Source: CAD feature listing. Evaluate the final solid. Frame: model axes, mm. A direction names the side the tool comes from. Give positions to 0.01 mm unless a question says otherwise; leave off trailing zeros. Write each loop counter-clockwise with the first axis right and the second up, starting at its lowest first coordinate (ties: lowest second). Pieces come first, ordered by that corner, then holes. Notation, with made-up numbers: (44, 9.25) -> (63, 9.25) arc R18 cw to (63, 42.25) -> close; hole circle Ø11 at (36.25, 76). An arc over 180 degrees is marked (long way). Write item = value, one per line.
from build123d import *

# Parameters (mm, degrees)
BOSS_EXTRUDE1_DEPTH             = 57.5
CUT_EXTRUDE1_DEPTH              = 334.110342079
CUT_EXTRUDE4_START              = 2.5
CUT_EXTRUDE4_DEPTH              = 322.334448445
BOSS_EXTRUDE2_REACH             = 325.834
SKETCH9_R                       = 5
BOSS_EXTRUDE2_DIRECTION_2_REACH = 325.834
CUT_EXTRUDE5_DEPTH              = 324.834448483
CUT_EXTRUDE5_DEPTH_BACK         = 324.834448483
SKETCH9_3_R                     = 5


with BuildPart() as part:
    # Sketch3 → Boss-Extrude1 (new, symmetric)
    with BuildSketch(Plane.YZ):
        with BuildLine():
            Line((242.818015058, -8.927876097), (206.857769199, 33.927876097))
            ThreePointArc((206.857769199, 33.927876097), (203.423507385, 36.56307787), (199.197324767, 37.5))
            Line((199.197324767, 37.5), (-37.5, 37.5))
            Line((-37.5, 37.5), (-37.5, -37.5))
            Line((-37.5, -37.5), (83.860297657, -37.5))
            ThreePointArc((83.860297657, -37.5), (87.280499091, -36.896926208), (90.288173754, -35.160444431))
            Line((90.288173754, -35.160444431), (126.423201987, -4.839555569))
            ThreePointArc((126.423201987, -4.839555569), (129.43087665, -3.103073792), (132.851078083, -2.5))
            Line((132.851078083, -2.5), (167.490945548, -2.5))
            ThreePointArc((167.490945548, -2.5), (171.717128165, -3.43692213), (175.151389979, -6.072123903))
            Line((175.151389979, -6.072123903), (219.50263215, -58.927876097))
            ThreePointArc((219.50263215, -58.927876097), (222.936893964, -61.56307787), (227.163076582, -62.5))
            Line((227.163076582, -62.5), (312.5, -62.5))
            Line((312.5, -62.5), (312.5, -12.5))
            Line((312.5, -12.5), (250.478459489, -12.5))
            ThreePointArc((250.478459489, -12.5), (246.252276872, -11.56307787), (242.818015058, -8.927876097))
        make_face()
    extrude(amount=BOSS_EXTRUDE1_DEPTH, both=True)

    # Sketch4 → Cut-Extrude1 (cut, through all)
    with BuildSketch(Plane.XY.offset(37.5)):
        Polygon((57.5, -37.5), (57.5, 37.5), (0, -37.5), align=None)
        Polygon((0, -37.5), (-57.5, 37.5), (-57.5, -37.5), align=None)
        Polygon((-37.232627886, 27.5), (0, -21.064297242), (0, 27.5), align=None)
        Polygon((0, 27.5), (0, -21.064297242), (37.232627886, 27.5), align=None)
        Polygon((57.5, 199.197324767), (38.166624213, 199.197324767), (57.5, 37.5), align=None)
        Polygon((-57.5, 37.5), (-38.166624213, 199.197324767), (-57.5, 199.197324767), align=None)
        Polygon((57.5, 312.5), (0, 312.5), (30, 267.5), (38.166624213, 199.197324767), (57.5, 199.197324767), (57.5, 250.478459489), align=None)
        Polygon((-30, 267.5), (0, 312.5), (-57.5, 312.5), (-57.5, 250.478459489), (-57.5, 199.197324767), (-38.166624213, 199.197324767), align=None)
        Polygon((0, 277.5), (0, 294.472243623), (-11.314829082, 277.5), align=None)
        Polygon((11.314829082, 277.5), (0, 294.472243623), (0, 277.5), align=None)
    extrude(amount=-CUT_EXTRUDE1_DEPTH, mode=Mode.SUBTRACT)

    # Sketch7 → Cut-Extrude4 (cut, through all)
    with BuildSketch(Plane.YZ.offset(CUT_EXTRUDE4_START)):
        with BuildLine():
            Line((37.5, 37.5), (37.5, -31.5))
            Line((37.5, -31.5), (83.860297657, -31.5))
            add(Edge.make_bspline(
                [(83.860297657, -31.5), (84.097540548, -31.5), (84.57337446, -31.458390238), (85.263019182, -31.273484118), (85.908338575, -30.972374338), (86.294621244, -30.70182834), (86.474686107, -30.55073598)],
                knots=[-1.570796327, -1.570796327, -1.570796327, -1.570796327, -1.396263402, -1.221730476, -1.047197551, -0.872664626, -0.872664626, -0.872664626, -0.872664626], degree=3))
            Line((86.474686107, -30.55073598), (122.609714339, -0.229847118))
            add(Edge.make_bspline(
                [(122.609714339, -0.229847118), (123.320382845, 0.366474563), (124.848442038, 1.436524541), (127.37869722, 2.615963904), (130.072824203, 3.338033288), (131.926306613, 3.5), (132.851078083, 3.5)],
                knots=[1.570796327, 1.570796327, 1.570796327, 1.570796327, 1.745329252, 1.919862177, 2.094395102, 2.268928028, 2.268928028, 2.268928028, 2.268928028], degree=3))
            Line((132.851078083, 3.5), (167.490945548, 3.5))
            add(Edge.make_bspline(
                [(167.490945548, 3.5), (168.646100732, 3.5), (170.964100646, 3.246604285), (174.273089477, 2.122910497), (177.265048317, 0.308445679), (178.955852245, -1.310444394), (179.701732038, -2.199349317)],
                knots=[0.698131701, 0.698131701, 0.698131701, 0.698131701, 0.916297857, 1.134464014, 1.35263017, 1.570796327, 1.570796327, 1.570796327, 1.570796327], degree=3))
            Line((179.701732038, -2.199349317), (224.052974209, -55.055101511))
            add(Edge.make_bspline(
                [(224.052974209, -55.055101511), (224.24085811, -55.279012825), (224.665398004, -55.685610911), (225.425771497, -56.147439629), (226.271617671, -56.434873066), (226.866794678, -56.5), (227.163076582, -56.5)],
                knots=[-2.443460953, -2.443460953, -2.443460953, -2.443460953, -2.225294796, -2.00712864, -1.788962483, -1.570796327, -1.570796327, -1.570796327, -1.570796327], degree=3))
            Line((227.163076582, -56.5), (267.5, -56.5))
            Line((267.5, -56.5), (267.5, -12.5))
            Line((267.5, -12.5), (250.478459489, -12.5))
            ThreePointArc((250.478459489, -12.5), (246.252276872, -11.56307787), (242.818015058, -8.927876097))
            Line((242.818015058, -8.927876097), (206.857769199, 33.927876097))
            ThreePointArc((206.857769199, 33.927876097), (203.423507385, 36.56307787), (199.197324767, 37.5))
            Line((199.197324767, 37.5), (37.5, 37.5))
        make_face()
    cut_extrude4 = extrude(amount=CUT_EXTRUDE4_DEPTH, mode=Mode.SUBTRACT)

    # Mirror1: Cut-Extrude4 across plane
    add(cut_extrude4.mirror(Plane(origin=(0, 0, 0), x_dir=(0, 0, 1), z_dir=(1, 0, 0))), mode=Mode.SUBTRACT)

    # Boss-Extrude2: up to this plane
    boss_extrude2_end = Plane(origin=(61.110075713, 7.306639487, -62.5), z_dir=(0.9929278168066742, 0.11871963027036327, 0))
    # Sketch9 → Boss-Extrude2 (add, up to the surface)
    with BuildSketch(Plane.YZ, mode=Mode.PRIVATE) as boss_extrude2_sk1:
        with BuildLine():
            Line((61.25, -17.5), (37.5, -17.5))
            Line((37.5, -17.5), (37.5, -37.5))
            Line((37.5, -37.5), (71.25, -37.5))
            Line((71.25, -37.5), (71.25, -27.5))
            ThreePointArc((71.25, -27.5), (68.321067812, -20.428932188), (61.25, -17.5))
        make_face()
        with Locations((61.25, -27.5)):
            Circle(SKETCH9_R, mode=Mode.SUBTRACT)
    boss_extrude2_tool1 = split(extrude(boss_extrude2_sk1.sketch, amount=BOSS_EXTRUDE2_REACH, mode=Mode.PRIVATE), bisect_by=boss_extrude2_end, keep=Keep.BOTH, mode=Mode.PRIVATE)
    add(boss_extrude2_tool1.solids().sort_by_distance((0, 52.889493, -27.789855))[0])
    # Sketch9 → Boss-Extrude2 (add, up to the surface)
    with BuildSketch(Plane.YZ, mode=Mode.PRIVATE) as boss_extrude2_sk2:
        with BuildLine():
            Line((267.5, -62.5), (267.5, -42.5))
            Line((267.5, -42.5), (252.5, -42.5))
            ThreePointArc((252.5, -42.5), (245.428932188, -45.428932188), (242.5, -52.5))
            Line((242.5, -52.5), (242.5, -62.5))
            Line((242.5, -62.5), (267.5, -62.5))
        make_face()
        with Locations((252.5, -52.5)):
            Circle(SKETCH9_R, mode=Mode.SUBTRACT)
    boss_extrude2_tool2 = split(extrude(boss_extrude2_sk2.sketch, amount=BOSS_EXTRUDE2_REACH, mode=Mode.PRIVATE), bisect_by=boss_extrude2_end, keep=Keep.BOTH, mode=Mode.PRIVATE)
    add(boss_extrude2_tool2.solids().sort_by_distance((0, 267.179844, -52.5))[0])

    # Boss-Extrude2 direction 2: up to this plane
    boss_extrude2_direction_2_end = Plane(origin=(-61.110075713, 7.306639487, -62.5), z_dir=(0.9929278168066742, -0.11871963027036327, 0))
    # Sketch9 → Boss-Extrude2 direction 2 (add, up to the surface)
    with BuildSketch(Plane.YZ, mode=Mode.PRIVATE) as boss_extrude2_direction_2_sk1:
        with BuildLine():
            Line((61.25, -17.5), (37.5, -17.5))
            Line((37.5, -17.5), (37.5, -37.5))
            Line((37.5, -37.5), (71.25, -37.5))
            Line((71.25, -37.5), (71.25, -27.5))
            ThreePointArc((71.25, -27.5), (68.321067812, -20.428932188), (61.25, -17.5))
        make_face()
        with Locations((61.25, -27.5)):
            Circle(SKETCH9_R, mode=Mode.SUBTRACT)
    boss_extrude2_direction_2_tool1 = split(extrude(boss_extrude2_direction_2_sk1.sketch, amount=-BOSS_EXTRUDE2_DIRECTION_2_REACH, mode=Mode.PRIVATE), bisect_by=boss_extrude2_direction_2_end, keep=Keep.BOTH, mode=Mode.PRIVATE)
    add(boss_extrude2_direction_2_tool1.solids().sort_by_distance((0, 52.889493, -27.789855))[0])
    # Sketch9 → Boss-Extrude2 direction 2 (add, up to the surface)
    with BuildSketch(Plane.YZ, mode=Mode.PRIVATE) as boss_extrude2_direction_2_sk2:
        with BuildLine():
            Line((267.5, -62.5), (267.5, -42.5))
            Line((267.5, -42.5), (252.5, -42.5))
            ThreePointArc((252.5, -42.5), (245.428932188, -45.428932188), (242.5, -52.5))
            Line((242.5, -52.5), (242.5, -62.5))
            Line((242.5, -62.5), (267.5, -62.5))
        make_face()
        with Locations((252.5, -52.5)):
            Circle(SKETCH9_R, mode=Mode.SUBTRACT)
    boss_extrude2_direction_2_tool2 = split(extrude(boss_extrude2_direction_2_sk2.sketch, amount=-BOSS_EXTRUDE2_DIRECTION_2_REACH, mode=Mode.PRIVATE), bisect_by=boss_extrude2_direction_2_end, keep=Keep.BOTH, mode=Mode.PRIVATE)
    add(boss_extrude2_direction_2_tool2.solids().sort_by_distance((0, 267.179844, -52.5))[0])

    # Sketch9_3 → Cut-Extrude5 (cut, two sides: drawn at the far end of the back side and taken through both)
    with BuildSketch(Plane.YZ.offset(-CUT_EXTRUDE5_DEPTH_BACK)):
        with Locations((61.25, -27.5)):
            Circle(SKETCH9_3_R)
        with Locations((252.5, -52.5)):
            Circle(SKETCH9_3_R)
    extrude(amount=CUT_EXTRUDE5_DEPTH + CUT_EXTRUDE5_DEPTH_BACK, mode=Mode.SUBTRACT)


solid = part.part
1) Cut plane A-A (y = -7.5). Return the cut outline in (x, z).
Computed:
outline = (-23, -37.5) -> (-10.4, -37.5) -> (-10.4, 37.5) -> (-23, 37.5) -> close; (10.4, -37.5) -> (23, -37.5) -> (23, 37.5) -> (10.4, 37.5) -> close
2) Cut plane B-B (y = 192). Return the cut outline in (x, z).
Computed:
outline = (-39.03, -26.15) -> (39.03, -26.15) -> (39.03, -16.86) -> (2.5, -16.86) -> (2.5, 37.5) -> (-2.5, 37.5) -> (-2.5, -16.86) -> (-39.03, -16.86) -> close
3) Draft query along Y for faces 1 (the flat face through (0, 275, -12.5)), 2 (the flat face through (-15, 290, -37)), 3 (the flat face through (-26.73, 104.29, -15.6)). Return one class per face: pulls with the +Y half, pulls with the -Y half, needs draft (parallel to the pull), parting line crosses it, or undercut.
Computed:
face_1 = needs draft
face_2 = pulls with the +Y half
face_3 = undercut
4) Contact query for flat-ended pins moving along their axis: pin 1 (12 mm diameter, centred on x = 11.5, y = 258.5, fed in from +Z); pin 2 (1 mm diameter, centred on x = 32.5, z = -11, fed in from -Y); pin 3 (2 mm diameter, centred on y = 248.5, z = -35, fed in from -X). Output: stop coordinate, or through.
Computed:
pin_1 = -42.5
pin_2 = 4.24
pin_3 = -2.5
5) Material intervals for L1, parallel to Z at x = 6, y = 252.5; L2, parallel to Z at x = -22, y = 61.25; L3, parallel to Y at x = 38, z = -15.5, sorted ascending.
Computed:
L1 = -62.5 to -57.5, -47.5 to -42.5
L2 = -37.5 to -32.5, -22.5 to -17.5
L3 = 12.07 to 37.5, 104.41 to 113.72, 183.06 to 190.86
6) Access query for faces 4 (the flat face through (-30, 50, -17.5)), 5 (the flat face through (0.04, 225.09, 12.2)), 6 (the flat face through (0.575, 197.017, -32.13)), 7 (the cylindrical face through (17.53, 245.51, -45.35)), 8 (the flat face through (-18.88, 3.56, 0.52)). Directions: +Z, -Z, +X, -X, +Y, -Y. A direction counts if a zero-diameter tool reaches every point of the face in a straight line with its end or side. Return the directions, or none.
Computed:
face_4 = +Z, -X
face_5 = +Z, +X, -X, +Y
face_6 = -Z, +X, -X
face_7 = +Z, +X
face_8 = +Z, -Z
